The figure shows three views and two pictorial views of one solid part (mm, origin at its lowest corner). Answer the questions. A direction names the side the tool comes from. Coordinates: 2 decimals unless noted, no trailing zeros. Order: outer loops, then holes, each group sorted by start corner. A loop starts at its lowest first (then second) coordinate and runs counter-clockwise, first axis right, second up. Notation, with made-up numbers: M -21.75,11.25 L 10.25,11.25 A28 ccw 10.25,39.25 Z; hole C 89,-5 d11. An arc over 180 degrees is marked long. Use a Markdown table: item, result.
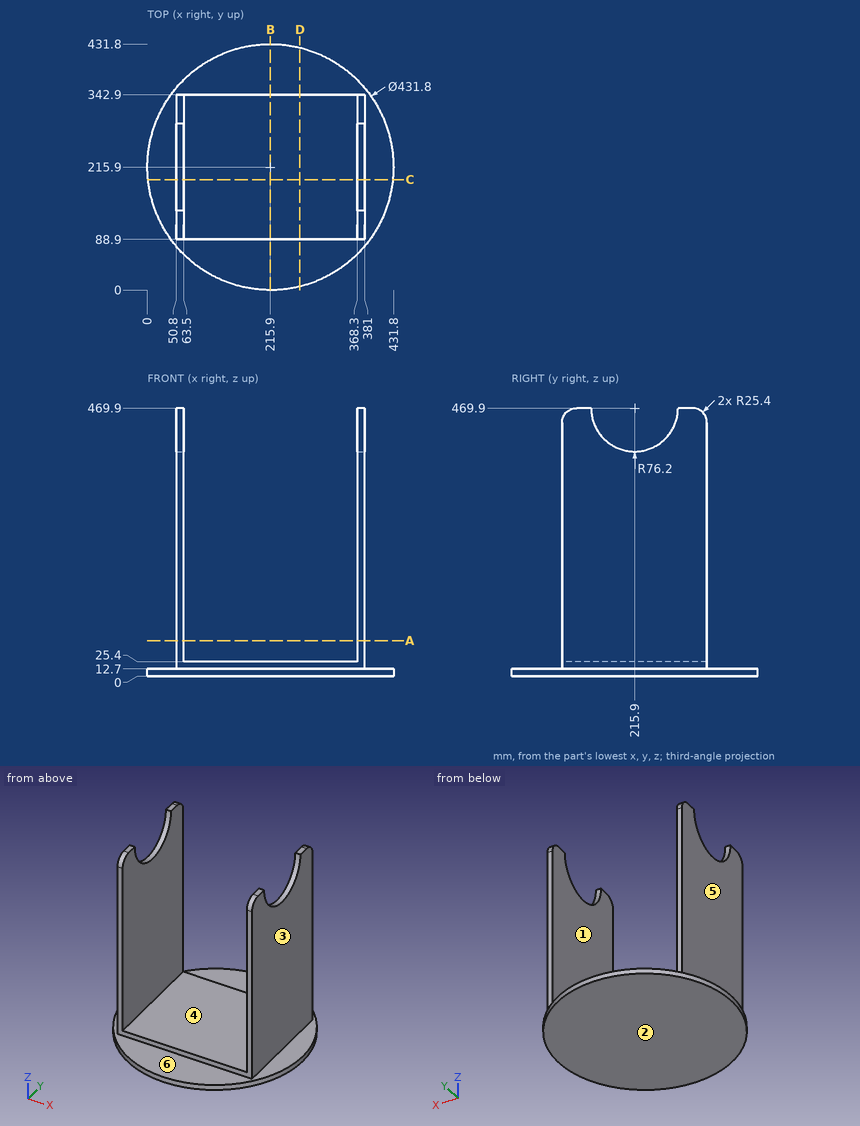
1. Section C-C on y = 194 is taken. Determine the outline of the cut face in (x, z), then the cut area to 3 significant figures.
Answers below:
| item | result |
|---|---|
| outline | M 1.11,0 L 430.69,0 L 430.69,12.7 L 381,12.7 L 381,396.91 L 368.3,396.91 L 368.3,25.4 L 63.5,25.4 L 63.5,396.91 L 50.8,396.91 L 50.8,12.7 L 1.11,12.7 Z |
| area | 19,100 mm² |
2. For a pull along X with two mould halves and no side action, classify the marked faces 4, 5 and 6 as +X half, -X half, draft (parallel to the pull), parting line (faces both ways), or undercut.
Answers below:
| item | result |
|---|---|
| face 4 | undercut |
| face 5 | -X half |
| face 6 | draft |
3. Find the intervals of material crossed by probe 1 along X at (y, z) = (177, 194.5); probe 2 along Z at (x, y) = (77.5, 103); probe 3 along Z at (x, y) = (255.5, 365), in increasing order.
Answers below:
| item | result |
|---|---|
| probe 1 | 50.8 to 63.5, 368.3 to 381 |
| probe 2 | 0 to 25.4 |
| probe 3 | 0 to 12.7 |
4. Section A-A on z = 62 is taken. Determine the outline of the cut face in (x, y), then the cut area to 3 significant figures.
Answers below:
| item | result |
|---|---|
| outline | M 50.8,88.9 L 63.5,88.9 L 63.5,342.9 L 50.8,342.9 Z; M 368.3,88.9 L 381,88.9 L 381,342.9 L 368.3,342.9 Z |
| area | 6,450 mm² |
5. Section D-D on x = 267.5 is taken. Determine the outline of the cut face in (y, z), then the cut area to 3 significant figures.
Answers below:
| item | result |
|---|---|
| outline | M 6.26,0 L 425.54,0 L 425.54,12.7 L 342.9,12.7 L 342.9,25.4 L 88.9,25.4 L 88.9,12.7 L 6.26,12.7 Z |
| area | 8,550 mm² |
6. For the marked faces 1, 2 and 3, determine the directions among +Z, -Z, +X, -X, +Y, -Y from which every point of the face is accessible in a straight line to the end or side of a thin tool.
Answers below:
| item | result |
|---|---|
| face 1 | +Z, +Y, -Y |
| face 2 | -Z, +X, -X, +Y, -Y |
| face 3 | +Z, +X, +Y, -Y |
7. Section B-B on x = 215.9 is taken. Determine the outline of the cut face in (y, z).
Answers below:
| item | result |
|---|---|
| outline | M 0,0 L 431.8,0 L 431.8,12.7 L 342.9,12.7 L 342.9,25.4 L 88.9,25.4 L 88.9,12.7 L 0,12.7 Z |
8. Flat-ended cylindrical pins translate along their axes: P1, Ø8, axis at y = 225, z = 232.5, coming from the -X side; P2, Ø5, axis at x = 331.5, y = 356.5, coming from the +Z side. Find the tip coordinate at first contact, or state that the pin passes through.
Answers below:
| item | result |
|---|---|
| P1 | x = 50.8 |
| P2 | z = 12.7 |
